from build123d import *

# Parameters (mm, degrees)
F1_DEPTH = 20
F2_R     = 7.5
F3_DEPTH = 15


with BuildPart() as f1:
    # F0 (on Top) → F1 (new body)
    with BuildSketch(Plane.XY):
        with BuildLine():
            Line((2, 3.75), (0, 3.75))
            Line((0, 3.75), (0, 0))
            Line((0, 0), (-2, 0))
            Line((-2, 0), (-2, -3))
            Line((-2, -3), (0, -3))
            Line((0, -3), (17.5, -3))
            ThreePointArc((17.5, -3), (28.106716, 1.092985), (33.214554, 11.25))
            Line((33.214554, 11.25), (33.214554, 28.71393))
            Line((33.214554, 28.71393), (23.58752, 28.71393))
            Line((23.58752, 28.71393), (23.58752, 22.71393))
            Line((23.58752, 22.71393), (26.58752, 22.71393))
            Line((26.58752, 22.71393), (26.58752, 25.75))
            Line((26.58752, 25.75), (30.33752, 25.75))
            Line((30.33752, 25.75), (30.33752, 11.25))
            ThreePointArc((30.33752, 11.25), (26.0347, 3.210474), (17.5, 0))
            Line((17.5, 0), (2, 0))
            Line((2, 0), (2, 3.75))
        make_face()
    extrude(amount=F1_DEPTH)

    # F2 (on face) → F3 (join)
    with BuildSketch(Plane.YZ.offset(33.214554)):
        with Locations((20.25, 10)):
            Circle(F2_R)
    extrude(amount=F3_DEPTH)


solid = f1.part
Here's how the part is built. I have some questions about the finished solid (model axes, mm). A direction names the side the tool comes from. Coordinates: 2 decimals unless noted, no trailing zeros. Order: outer loops, then holes, each group sorted by start corner. A loop starts at its lowest first (then second) coordinate and runs counter-clockwise, first axis right, second up. Notation, with made-up numbers: M 84.5,13 L 97.5,13 A21 ccw 97.5,26 Z; hole C 4,76 d8. An arc over 180 degrees is marked long. Answer as CSV lines item,"result". Start each with the question number.
1. On a 3-axis mill with a long thin cutter (end or side, diameter ignored), from which of +Z, -Z, +X, -X, +Y, -Y can I reach the whole of each face in a straight line? I mean faces 1 (the flat face through (30.338, 19, 10)), 2 (the flat face through (2, 2, 10)), 3 (the cylindrical face through (40.61, 14.298, 5.436)), 4 (the flat face through (-1, 0, 10)). Say none if no direction works.
2. For pin 1 (5 mm diameter, centred on y = 10.5, z = 5, fed in from +X); pin 2 (3 mm diameter, centred on y = 25.5, z = 10.5, fed in from -X); pin 3 (1 mm diameter, centred on x = -1.5, z = 8, fed in from +Y); pin 4 (8 mm diameter, centred on x = 16.5, y = 23, fed in from -Z), each with a flat end and sliding along its axis, tell me the tip position at first contact or that it passes through.
3. I want a section at C-C, the plane y = 20.25. Write out the boundary of the cut face in (x, z).
4. We'd pull the mould along Y, two halves only. Please class faces 5 (the flat face through (10, 0, 10)), 6 (the flat face through (28, 25.75, 10)), 7 (the flat face through (23.588, 26, 10)), 8 (the flat face through (26.588, 24, 10)): released by +Y, released by -Y, zero draft, split by the parting line, or undercut.
5. I want a section at A-A, the plane y = 1.5. Write out the boundary of the cut face in (x, z), and give its area (3 significant figures).
6. I want a section at B-B, the plane z = 10. Write out the boundary of the cut face in (x, y).
7. I need wall thicknesses on line 1 (X direction, y = 25.5, z = 1.5); line 2 (X direction, y = 25.5, z = 12.75); line 3 (X direction, y = 18, z = 17.25). Which ranges of each line are inside material? Lowest first, please. Write a range as [from, to].
8. I want a section at D-D, the plane x = 7. Write out the boundary of the cut face in (y, z), and give its area (3 significant figures).
Recorded:
1,face 1,"+Z, -Z"
1,face 2,"+Z, -Z, +Y"
1,face 3,"+X"
1,face 4,"+Z, -Z, -X, +Y"
2,pin 1,"stops at x = 33.21"
2,pin 2,"stops at x = 23.59"
2,pin 3,"stops at y = 0"
2,pin 4,"passes through"
3,outline,"M 30.34,0 L 33.21,0 L 33.21,2.5 L 48.21,2.5 L 48.21,17.5 L 33.21,17.5 L 33.21,20 L 30.34,20 Z"
4,face 5,"released by +Y"
4,face 6,"undercut"
4,face 7,"zero draft"
4,face 8,"undercut"
5,outline,"M 0,0 L 2,0 L 2,20 L 0,20 Z; M 23.55,0 L 28.54,0 L 28.54,20 L 23.55,20 Z"
5,area,"140 mm2"
6,outline,"M -2,-3 L 17.5,-3 A15.79 ccw 33.21,11.25 L 33.21,12.75 L 48.21,12.75 L 48.21,27.75 L 33.21,27.75 L 33.21,28.71 L 23.59,28.71 L 23.59,22.71 L 26.59,22.71 L 26.59,25.75 L 30.34,25.75 L 30.34,11.25 A12.95 cw 17.5,0 L 2,0 L 2,3.75 L 0,3.75 L 0,0 L -2,0 Z"
7,line 1,"x = [23.59, 26.59], [30.34, 33.21]"
7,line 2,"x = [23.59, 26.59], [30.34, 48.21]"
7,line 3,"x = [30.34, 33.21]"
8,outline,"M -3,0 L 0,0 L 0,20 L -3,20 Z"
8,area,"60.0 mm2"
